The listing builds one solid part. Answer for the finished solid, in the listing's coordinates (mm). Face numbers are marked on the shaded views. A direction names the side the tool comes from. Coordinates: 2 decimals unless noted, no trailing zeros. Loops run counter-clockwise (first coordinate to the right, second up) from the corner with the lowest first, then second, coordinate; pieces in that order, holes last. Notation, with made-up numbers: M -21.5,41.5 L 2.5,41.5 A31 ccw 2.5,73.5 Z; hole C 78.5,10 d3. An arc over 180 degrees is marked long. Return JSON: item names as keys, results as strings. Group by question number.
1. Section D-D (y = -1) is taken. Write down the section's boundary in (x, z).
2. Given P1, Ø5, axis at y = 17.5, z = -3, coming from the -X side; P2, Ø5.5, axis at x = -0.5, y = 30, coming from the -Z side; P3, Ø1.8, axis at y = 8.5, z = 20.5, coming from the +X side; P4, Ø3.5, axis at x = 0.5, z = 18.5, coming from the +Y side (3 decimals), each flat-ended and moving along its own axis, determine where each tip first touches the part or whether it passes through.
3. Section A-A (z = 0) is taken. Write down the section's boundary in (x, y) (3 decimals).
4. Section B-B (x = 0) is taken. Write down the section's boundary in (y, z) (1 decimal).
5. Section C-C (y = 10) is taken. Write down the section's boundary in (x, z).
6. The mould has two halves that part along Z. Classify the marked faces 5, 6, 7 and 8: pulls with the +Z half, pulls with the -Z half, needs draft (parallel to the pull), parting line crosses it, or undercut.
7. Which of the six approach directions +Z, -Z, +X, -X, +Y, -Y give full straight-line access (tool end or side, diameter ignored) to the marked faces 1, 2, 3 and 4?
8. Straight lines are drawn through the part: L1, parallel to X at y = 22, z = 0; L2, parallel to Y at x = 15.5, z = -2.5 (3 decimals); L3, parallel to X at y = 17, z = -3.5. For each, find the intervals that lie inside material, in ascending order. Write a range as from..to.
```python
from build123d import *

# Parameters (mm, degrees)
SKETCH2_R           = 17.5
BOSS_EXTRUDE1_DEPTH = 32.665
SKETCH3_R           = 12.5
BOSS_EXTRUDE2_DEPTH = 15
SKETCH4_R           = 13
CUT_EXTRUDE1_DEPTH  = 25
SKETCH8_W           = 35
SKETCH8_H           = 1.857450862
CUT_EXTRUDE4_DEPTH  = 35
SKETCH11_W          = 35
SKETCH11_H          = 2.234434129
CUT_EXTRUDE8_DEPTH  = 35
SKETCH13_W          = 5.276362384
SKETCH13_H          = 6.1175
BOSS_EXTRUDE3_DEPTH = 6.1175
SKETCH14_W          = 5.276362384
SKETCH14_H          = 6.1175
BOSS_EXTRUDE4_DEPTH = 6.1175
SKETCH18_R          = 0.79375
CUT_EXTRUDE11_DEPTH = 6.1175
SKETCH15_R          = 0.79375
CUT_EXTRUDE12_DEPTH = 6.1175
FILLET8_R           = 3.06
FILLET9_R           = 3.06
FILLET10_R          = 3.06
FILLET11_R          = 3.06


with BuildPart() as part:
    # Sketch2 → Boss-Extrude1 (new body)
    with BuildSketch(Plane(origin=(0, 0, 0), x_dir=(1, 0, 0), z_dir=(0, 1, 0))):
        with Locations(Location((0, 0, 0), (0, 0, 270))):
            Circle(SKETCH2_R)
    extrude(amount=BOSS_EXTRUDE1_DEPTH)

    # Sketch3 → Boss-Extrude2 (add)
    with BuildSketch(Plane.XZ):
        with Locations(Location((0, 0, 0), (0, 0, 270))):
            Circle(SKETCH3_R)
    extrude(amount=BOSS_EXTRUDE2_DEPTH)

    # Sketch4 → Cut-Extrude1 (cut)
    with BuildSketch(Plane(origin=(0, 32.665, 0), x_dir=(1, 0, 0), z_dir=(0, 1, 0))):
        with Locations(Location((0, 0, 0), (0, 0, 270))):
            Circle(SKETCH4_R)
    extrude(amount=-CUT_EXTRUDE1_DEPTH, mode=Mode.SUBTRACT)

    # Sketch8 → Cut-Extrude4 (cut)
    with BuildSketch(Plane(origin=(0, 32.665, 0), x_dir=(1, 0, 0), z_dir=(0, 1, 0))):
        with Locations((0, -18.228725431)):
            Rectangle(SKETCH8_W, SKETCH8_H)
    extrude(amount=-CUT_EXTRUDE4_DEPTH, mode=Mode.SUBTRACT)

    # Sketch11 → Cut-Extrude8 (cut)
    with BuildSketch(Plane(origin=(0, 32.665, 0), x_dir=(1, 0, 0), z_dir=(0, 1, 0))):
        with Locations((0, 18.417217065)):
            Rectangle(SKETCH11_W, SKETCH11_H)
    extrude(amount=-CUT_EXTRUDE8_DEPTH, mode=Mode.SUBTRACT)

    # Sketch13 → Boss-Extrude3 (add)
    with BuildSketch(Plane(origin=(0, 0, -17.3), x_dir=(-1, 0, 0), z_dir=(0, 0, -1))):
        with Locations((0, 24.60625)):
            Rectangle(SKETCH13_W, SKETCH13_H)
    extrude(amount=BOSS_EXTRUDE3_DEPTH)

    # Sketch14 → Boss-Extrude4 (add)
    with BuildSketch(Plane.XY.offset(17.3)):
        with Locations((0, 8.05875)):
            Rectangle(SKETCH14_W, SKETCH14_H)
    extrude(amount=BOSS_EXTRUDE4_DEPTH)

    # Sketch18 → Cut-Extrude11 (cut)
    with BuildSketch(Plane(origin=(2.638181192, 0, 0), x_dir=(0, 0, -1), z_dir=(1, 0, 0))):
        with Locations((-19.565, 8.0575)):
            Circle(SKETCH18_R)
    extrude(amount=-CUT_EXTRUDE11_DEPTH, mode=Mode.SUBTRACT)

    # Sketch15 → Cut-Extrude12 (cut)
    with BuildSketch(Plane(origin=(2.638181192, 0, 0), x_dir=(0, 0, -1), z_dir=(1, 0, 0))):
        with Locations(Location((19.565, 24.60625, 0), (0, 0, 90))):
            Circle(SKETCH15_R)
    extrude(amount=-CUT_EXTRUDE12_DEPTH, mode=Mode.SUBTRACT)

    # Fillet8
    fillet8_edges = [part.edges().sort_by_distance(p)[0] for p in [
        (0, 27.665, -23.4175),
    ]]
    fillet(fillet8_edges, radius=FILLET8_R)

    # Fillet9
    # the kernel refuses this fillet: 3.06 mm, written as the material it takes off along each edge
    with BuildSketch(Plane(origin=(-10.288181192, 21.5475, -23.4175), x_dir=(0, 1, 0), z_dir=(1, 0, 0))) as fillet9_piece_1:
        with BuildLine():
            CenterArc((FILLET9_R, FILLET9_R), FILLET9_R, 180, 90)
            Line((0, FILLET9_R), (0, 0))
            Line((0, 0), (FILLET9_R, 0))
        make_face()
    extrude(amount=20.576362383, mode=Mode.SUBTRACT)

    # Fillet10
    fillet10_edges = [part.edges().sort_by_distance(p)[0] for p in [
        (0, 11.1175, 23.4175),
    ]]
    fillet(fillet10_edges, radius=FILLET10_R)

    # Fillet11
    # the kernel refuses this fillet: 3.06 mm, written as the material it takes off along each edge
    with BuildSketch(Plane(origin=(10.288181192, 5, 23.4175), x_dir=(0, 1, 0), z_dir=(-1, 0, 0))) as fillet11_piece_1:
        with BuildLine():
            CenterArc((FILLET11_R, FILLET11_R), FILLET11_R, 180, 90)
            Line((0, FILLET11_R), (0, 0))
            Line((0, 0), (FILLET11_R, 0))
        make_face()
    extrude(amount=20.576362383, mode=Mode.SUBTRACT)


solid = part.part
```
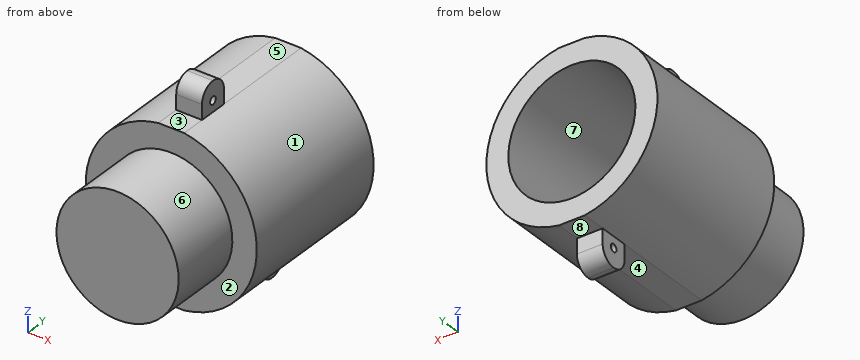
Worked out:
{
 "1": {"outline": "C 0,0 d25"},
 "2": {"P1": "x = -17.49", "P2": "z = -21.9", "P3": "x = 2.64", "P4": "y = 32.665"},
 "3": {"outline": "M -17.5,0 L -12.5,0 L -12.5,-15 L 12.5,-15 L 12.5,0 L 17.5,0 L 17.5,32.665 L 13,32.665 L 13,7.665 L -13,7.665 L -13,32.665 L -17.5,32.665 Z"},
 "4": {"outline": "M -15,-12.5 L 0,-12.5 L 0,-17.3 L 21.5,-17.3 L 21.5,-20.4 A3.1 ccw 24.6,-23.4 A3.1 ccw 27.7,-20.4 L 27.7,-17.3 L 32.7,-17.3 L 32.7,-13 L 7.7,-13 L 7.7,13 L 32.7,13 L 32.7,17.3 L 11.1,17.3 L 11.1,20.4 A3.1 ccw 8.1,23.4 A3.1 ccw 5,20.4 L 5,17.3 L 0,17.3 L 0,12.5 L -15,12.5 Z; hole C 8.1,19.6 d1.6; hole C 24.6,-19.6 d1.6"},
 "5": {"outline": "M -2.64,-17.3 L 2.64,-17.3 A17.5 ccw 2.64,17.3 L 2.64,22.72 L -2.64,22.72 L -2.64,17.3 A17.5 ccw Z; hole C 0,0 d26"},
 "6": {"face 5": "pulls with the +Z half", "face 6": "parting line crosses it", "face 7": "undercut", "face 8": "pulls with the -Z half"},
 "7": {"face 1": "+X, +Y, -Y", "face 2": "-Y", "face 3": "+Z, +X, -X, -Y", "face 4": "-Z, +X, -X, -Y"},
 "8": {"L1": "-17.5..-13, 13..17.5", "L2": "0..32.665", "L3": "-17.15..-12.52, 12.52..17.15"}
}
